The model under review builds one solid part; all positions refer to its coordinate system, in mm. A direction names the side the tool comes from. Coordinates: 2 decimals unless noted, no trailing zeros. Loops run counter-clockwise (first coordinate to the right, second up) from the corner with the lowest first, then second, coordinate; pieces in that order, holes last. Notation, with made-up numbers: (61.25, 32) - (70.25, 32) arc R23 cw to (70.25, 49) - close; hole circle Ø11 at (55.5, 29.5). An arc over 180 degrees is marked (long way). Answer in a Markdown table with one row per item. Add a question column.
(1) Mouldability with a two-part tool opening along Z and no side actions: class faces 1 (the flat face through (0, 3, -56)), 2 (the flat face through (0, 13, -67.295)), 3 (the flat face through (56, 25, 1)) as +Z half, -Z half, draft (parallel to the pull), parting line (faces both ways), or undercut.
(2) We need section D-D on z = -31. Write out the cut boundary in (x, y), plus the area to 3 significant figures.
(3) We need section A-A on x = 0. Write out the cut boundary in (y, z) (3 decimals), plus the area to 3 significant figures.
(4) For line 1 along Z through (x, y) = (0, 0.75) (3 decimals); line 2 along Y through (x, z) = (35, -7.5); line 3 along X through (y, z) = (13.25, -28), list the stretches that pass through material, from the lowest coordinate up.
(5) We need section B-B on y = 22.5. Write out the cut boundary in (x, z) (1 decimal).
(6) Machinability: for faces 4 (the flat face through (9.924, 12, -62)), 5 (the flat face through (0, 3, 0)), 6 (the flat face through (67, 23, 57.295)), which of the approach directions +Z, -Z, +X, -X, +Y, -Y give a long, thin tool a straight path to every point of the face, cutting with its end or side? Answer none if there is none.
(7) We need section C-C on z = 0. Write out the cut boundary in (x, y).
(8) For P1, Ø3, axis at y = 12, z = -60.5, coming from the +X side; P2, Ø3.5, axis at x = 1, z = 57.5, coming from the -Y side; P3, Ø12, axis at x = 48, y = 22.5, coming from the +Z side (3 decimals), all flat-tipped, find the tip position at first contact; note any pin that passes through.
Autodesk Inventor part; units mm, degrees
ref_plane "YZ Plane" through (0, 0, 0) normal (1, 0, 0) x (0, 1, 0)
ref_plane "XZ Plane" through (0, 0, 0) normal (0, 1, 0) x (-1, 0, 0)
ref_plane "XY Plane" through (0, 0, 0) normal (0, 0, 1) x (1, 0, 0)
sketch "Sketch1" plane through (0, 0, 0) normal (0, 1, 0) x (-1, 0, 0)
  line L0 (10, -57.295) -> (-10, -57.295)
  line L1 (-10, -57.295) -> (-10, 57.295)
  line L2 (-10, 57.295) -> (10, 57.295)
  line L3 (10, 57.295) -> (10, -57.295)
  line L4 (10, -57.295) -> (-10, 57.295) construction
  line L5 (-10, -57.295) -> (10, 57.295) construction
  point P0 (0, 0)
  dimension "d0" = 114.59
  dimension "d1" = 20
extrude "Extrusion1" add sketch "Sketch1" along normal blind 25
sketch "Sketch2" plane through (10, 0, 57.295) normal (1, 0, 0) x (0, 0, -1)
  line L0 (0, 0) -> (0, 25)
  line L1 (114.59, 0) -> (114.59, 25)
  line L2 (0, 25) -> (114.59, 25)
  line L3 (114.59, 25) -> (114.59, 20.6952)
  line L4 (114.59, 20.6952) -> (0, 20.6952)
  line L5 (0, 20.6952) -> (0, 25)
  point P0 (57.295, 0)
extrude "Extrusion2" add sketch "Sketch2" along normal blind 114
sketch "Sketch3" plane through (0, 0, 0) normal (0, -1, 0) x (1, 0, 0)
  circle A0 centre (0, 0) radius 6
  circle A1 centre (0, -56.1484) radius 6
  circle A2 centre (0, 56.972) radius 6
  dimension "d7" = 12
  dimension "d9" = 12
  dimension "d10" = 12
sketch "Sketch4" plane through (-10, 0, 57.295) normal (0, 0, 1) x (1, 0, 0)
  line L0 (20, 0) -> (0, 0)
  line L1 (0, 25) -> (134, 25)
  line L2 (0, 0) -> (19.9687, 0)
  line L3 (19.9687, 0) -> (19.9687, 25)
  line L4 (19.9687, 25) -> (0, 25)
  line L5 (0, 25) -> (0, 0)
  point P0 (10, 0)
  point P1 (0, 25)
extrude "Extrusion3" add sketch "Sketch4" along normal blind 10
sketch "Sketch5" plane through (10, 0, -57.295) normal (0, 0, -1) x (-1, 0, 0)
  line L0 (20, 0) -> (20, 25)
  line L1 (20, 25) -> (-114, 25)
  line L2 (20, 0) -> (0.0765, 0)
  line L3 (0.0765, 0) -> (0.0765, 25)
  line L4 (0.0765, 25) -> (20, 25)
  line L5 (20, 25) -> (20, 0)
  point P0 (10, 0)
extrude "Extrusion4" add sketch "Sketch5" along normal blind 10
extrude "Extrusion5" cut sketch "Sketch3" against normal blind 3
properties part number "compartment 1"
Outcome:
| question | item | result |
|---|---|---|
| 1 | face 1 | undercut |
| 1 | face 2 | -Z half |
| 1 | face 3 | draft |
| 2 | outline | (-10, 0) - (10, 0) - (10, 20.7) - (124, 20.7) - (124, 25) - (-10, 25) - close |
| 2 | area | 991 mm² |
| 3 | outline | (0, -67.295) - (25, -67.295) - (25, 67.295) - (0, 67.295) - (0, 62.972) - (3, 62.972) - (3, 50.972) - (0, 50.972) - (0, 6) - (3, 6) - (3, -6) - (0, -6) - (0, -50.148) - (3, -50.148) - (3, -62.148) - (0, -62.148) - close |
| 3 | area | 3,260 mm² |
| 4 | line 1 | -67.295 to -62.148, -50.148 to -6, 6 to 50.972, 62.972 to 67.295 |
| 4 | line 2 | 20.7 to 25 |
| 4 | line 3 | -10 to 10 |
| 5 | outline | (-10, -67.3) - (9.9, -67.3) - (9.9, -57.3) - (124, -57.3) - (124, 57.3) - (10, 57.3) - (10, 67.3) - (-10, 67.3) - close |
| 6 | face 4 | -Z, +X, +Y, -Y |
| 6 | face 5 | -Y |
| 6 | face 6 | +Z, +X, +Y, -Y |
| 7 | outline | (-10, 0) - (-6, 0) - (-6, 3) - (6, 3) - (6, 0) - (10, 0) - (10, 20.7) - (124, 20.7) - (124, 25) - (-10, 25) - close |
| 8 | P1 | x = 9.92 |
| 8 | P2 | y = 3 |
| 8 | P3 | z = 57.295 |
